Input: part model. Units: mm. Frame: model coordinates. Face numbers are marked on the shaded views. A direction names the side the tool comes from. Round coordinates to 2 decimals unless told otherwise and drop trailing zeros. Loops run counter-clockwise (first coordinate to the right, second up) from the corner with the lowest first, then second, coordinate; pieces in that order, holes last. Notation, with made-up numbers: (6, -26) -> (14, -26) arc R11 cw to (14, -17) -> close; hole circle Ø6 at (33, 80). An arc over 180 degrees is marked (long way). Answer as a JSON object with one key per item and string values.
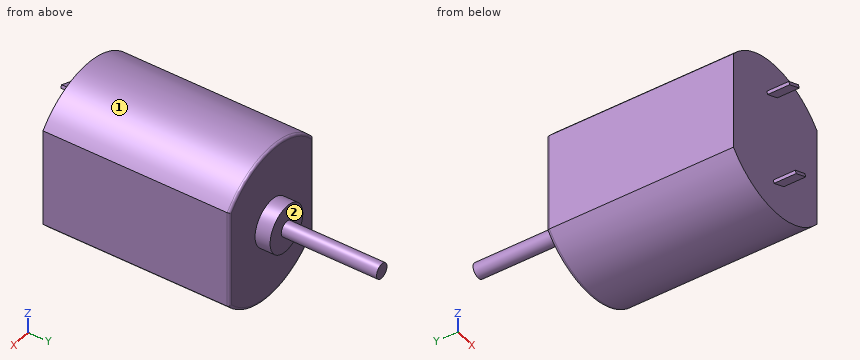
```python
from build123d import *

# Parameters (mm, degrees)
BOSS_EXTRUDE1_DEPTH = 18.6
BOSS_EXTRUDE2_DEPTH = 2.2
SKETCH3_R           = 2.35
BOSS_EXTRUDE3_DEPTH = 1.5
SKETCH4_R           = 0.75
BOSS_EXTRUDE4_DEPTH = 9.5
FILLET2_R           = 0.25


with BuildPart() as part:
    # Sketch1 → Boss-Extrude1 (new body)
    with BuildSketch(Plane(origin=(0, 0, 0), x_dir=(1, 0, 0), z_dir=(0, 1, 0))):
        with BuildLine():
            Line((-6, 4.983974318), (-6, -4.983974318))
            ThreePointArc((-6, -4.983974318), (0, -7.8), (6, -4.983974318))
            Line((6, -4.983974318), (6, 4.983974318))
            ThreePointArc((6, 4.983974318), (0, 7.8), (-6, 4.983974318))
        make_face()
    extrude(amount=BOSS_EXTRUDE1_DEPTH)

    # Sketch2 → Boss-Extrude2 (add)
    with BuildSketch(Plane.XZ):
        Polygon((1.212939296, -4.265123476), (1.095719957, -3.98897202), (-0.285037323, -4.575068713), (-0.167817984, -4.851220169), align=None)
        Polygon((0.285037323, 4.575068713), (0.167817984, 4.851220169), (-1.212939296, 4.265123476), (-1.095719957, 3.98897202), align=None)
    extrude(amount=BOSS_EXTRUDE2_DEPTH)

    # Sketch3 → Boss-Extrude3 (add)
    with BuildSketch(Plane(origin=(0, 18.6, 0), x_dir=(1, 0, 0), z_dir=(0, 1, 0))):
        with Locations(Location((0, 0, 0), (0, 0, 270))):
            Circle(SKETCH3_R)
    extrude(amount=BOSS_EXTRUDE3_DEPTH)

    # Sketch4 → Boss-Extrude4 (add)
    with BuildSketch(Plane(origin=(0, 20.1, 0), x_dir=(1, 0, 0), z_dir=(0, 1, 0))):
        with Locations(Location((0, 0, 0), (0, 0, 270))):
            Circle(SKETCH4_R)
    extrude(amount=BOSS_EXTRUDE4_DEPTH)

    # Fillet2
    fillet2_edges = [part.edges().sort_by_distance(p)[0] for p in [
        (0, 18.6, 7.8),
        (6, 18.6, 0),
        (0, 18.6, -7.8),
        (-6, 18.6, 0),
    ]]
    fillet(fillet2_edges, radius=FILLET2_R)


solid = part.part
```
1) Ray query, probe 1 along Y at (x, z) = (-2.5, -1.5); probe 2 along Y at (x, z) = (0.5, 2); probe 3 along Z at (x, y) = (3.25, 1). Return the intervals inside material, ascending.
Output:
{"probe 1": "y = 0 to 18.6", "probe 2": "y = 0 to 20.1", "probe 3": "z = -7.09 to 7.09"}
2) Section B-B, the plane y = 19.5. Output: boundary loops of the cut face in (x, z), plus the area to 3 significant figures.
Output:
{"outline": "circle Ø4.7 at (0, 0)", "area": "17.3 mm^2"}
3) Reachability of the marked faces 1 and 2 from +Z, -Z, +X, -X, +Y, -Y: full face, straight path, thin tool, end or side. Return the list, or none.
Output:
{"face 1": "+Z, +Y, -Y", "face 2": "+Y"}
4) Contact query for flat-ended pins moving along their axis: P1, Ø3.5, axis at x = 2, z = 3, coming from the -Y side; P2, Ø2, axis at x = -0.5, z = 3, coming from the +Y side; P3, Ø1.5, axis at x = 4.5, y = 3.5, coming from the -Z side. Output: stop coordinate, or through.
Output:
{"P1": "stops at y = 0", "P2": "stops at y = 20.1", "P3": "stops at z = -6.84"}
5) Section C-C, the plane y = 7. Output: boundary loops of the cut face in (x, z).
Output:
{"outline": "(-6, -4.98) arc R7.8 ccw to (6, -4.98) -> (6, 4.98) arc R7.8 ccw to (-6, 4.98) -> close"}
6) Section A-A, the plane z = 0. Output: boundary loops of the cut face in (x, y), plus the area to 3 significant figures.
Output:
{"outline": "(-6, 0) -> (6, 0) -> (6, 18.35) arc R0.25 ccw to (5.75, 18.6) -> (2.35, 18.6) -> (2.35, 20.1) -> (0.75, 20.1) -> (0.75, 29.6) -> (-0.75, 29.6) -> (-0.75, 20.1) -> (-2.35, 20.1) -> (-2.35, 18.6) -> (-5.75, 18.6) arc R0.25 ccw to (-6, 18.35) -> close", "area": "244 mm^2"}
